Autodesk Inventor part; units mm, degrees
ref_plane "Work Plane5" through (4.6312, 3.8939, 0) normal (1, 0, 0) x (0, 0, -1)
ref_plane "YZ Plane" through (0, 0, 0) normal (1, 0, 0) x (0, 1, 0)
ref_plane "XZ Plane" through (0, 0, 0) normal (0, 1, 0) x (-1, 0, 0)
sketch "Sketch1" plane through (0, 0, 0) normal (0, 0, 1) x (1, 0, 0)
  line L0 (0, 0) -> (9.3091, 0)
  line L1 (9.3091, 0) -> (9.3091, 10)
  line L2 (9.3091, 10) -> (0, 10)
  line L3 (0, 10) -> (0, 0)
  circle A0 centre (4.6631, 6.6706) radius 2.3
  circle A1 centre (4.6631, 6.6706) radius 1
  line L4 (4.6312, 3.0206) -> (4.6312, 4.3708)
  line L5 (4.6312, 8.9703) -> (4.6312, 9.9704)
  arc A2 (4.6312, 9.9704) -> (1.3632, 6.6438) centre (4.6631, 6.6706) ccw
  arc A3 (4.639, 4.4786) -> (4.6548, 4.4787) centre (4.6389, 7.7786) ccw
  arc A4 (0, 0) -> (1.3632, 6.6438) centre (-14.8677, 6.5123) ccw
  arc A5 (0, 0) -> (4.6312, 3.0206) centre (0.3336, 4.5492) ccw
  dimension "d0" = 10
  dimension "d1" = 4.6
  dimension "d2" = 2
extrude "Extrusion1" add sketch "Sketch1" along normal blind 4 contours A4 A2 L5 A0 L4 A5 L0 | L0 A5 | A0
fillet "Fillet1" radius 2 1 edges at (4.6312, 3.0206, 2)
sketch "Sketch2" plane through (0, 0, 4) normal (0, 0, 1) x (1, 0, 0)
  line L0 (4.6312, 3.4171) -> (4.6312, 4.3708)
  arc A0 (4.6312, 4.3708) -> (4.6312, 8.9703) centre (4.6631, 6.6706) ccw
  line L1 (4.6312, 8.9703) -> (4.6312, 9.9704)
  arc A1 (4.6312, 9.9704) -> (1.3632, 6.6438) centre (4.6631, 6.6706) ccw
  circle A2 centre (4.6631, 6.6706) radius 1
  circle A3 centre (4.6631, 6.6706) radius 2.3
  arc A4 (4.4253, 2.5332) -> (4.6312, 3.4171) centre (2.6312, 3.4171) ccw
  arc A5 (0, 0) -> (1.3632, 6.6438) centre (-14.8677, 6.5123) ccw
  arc A6 (0, 0) -> (4.4253, 2.5332) centre (0.3336, 4.5492) ccw
extrude "Extrusion2" cut sketch "Sketch2" against normal blind 1.3 contours A3 A0
sketch "Sketch3" plane through (0, 0, 0) normal (0, 0, -1) x (-1, 0, 0)
  arc A0 (-1.3632, 6.6438) -> (-4.6312, 9.9704) centre (-4.6631, 6.6706) ccw
  line L0 (-4.6312, 8.9703) -> (-4.6312, 9.9704)
  arc A1 (-4.6312, 8.9703) -> (-4.6312, 4.3708) centre (-4.6631, 6.6706) ccw
  line L1 (-4.6312, 3.4171) -> (-4.6312, 4.3708)
  circle A2 centre (-4.6631, 6.6706) radius 1
  circle A3 centre (-4.6631, 6.6706) radius 2.3
  arc A4 (-4.6312, 3.4171) -> (-4.4253, 2.5332) centre (-2.6312, 3.4171) ccw
  arc A5 (-4.4253, 2.5332) -> (0, 0) centre (-0.3336, 4.5492) ccw
  arc A6 (-1.3632, 6.6438) -> (0, 0) centre (14.8677, 6.5123) ccw
extrude "Extrusion3" cut sketch "Sketch3" against normal blind 1.3 contours A3 A1
ref_plane "Work Plane5" through (4.6312, 3.8939, 0) normal (1, 0, 0) x (0, 0, -1)
sketch "Sketch6" plane through (4.6312, 3.8939, 0) normal (1, 0, 0) x (0, 0, -1)
  line L0 (0, -0.4768) -> (0, 0.4768)
  line L1 (0, 0.4768) -> (-1.3, 0.4768)
  line L2 (-1.3, 0.4768) -> (-2.7, 0.4768)
  line L3 (-2.7, 0.4768) -> (-4, 0.4768)
  line L4 (-4, -0.4768) -> (-4, 0.4768)
  circle A0 centre (-2, 0.1418) radius 0.275
  line L5 (-4, -0.4768) -> (-4, 0.4768)
  line L6 (0, -0.4768) -> (-4, -0.4768)
  line L7 (0, -0.4768) -> (0, 0.4768)
  line L8 (-4, 0.4768) -> (0, 0.4768)
  line L9 (0, 0.4768) -> (0, -0.1932)
  line L10 (0, -0.1932) -> (-4, -0.1932)
  line L11 (-4, -0.1932) -> (-4, 0.4768)
  line L12 (-4, 0.4768) -> (0, -0.1932) construction
  line L13 (-4, -0.1932) -> (0, 0.4768) construction
  point P0 (0, -3.8939)
  dimension "d22" = 0.55
  dimension "d26" = 0.67
extrude "Extrusion6" cut sketch "Sketch6" against normal blind 0.475 contours A0
fillet "Fillet2" radius 0.3 1 edges at (0, 0, 2)
properties material "Liga de Nickel-Copper 400"
The model under review builds one solid part; all positions refer to its coordinate system, in mm. A direction names the side the tool comes from. Round coordinates to 2 decimals unless told otherwise and drop trailing zeros. Write each loop counter-clockwise with the first axis right and the second up, starting at its lowest first coordinate (ties: lowest second). Pieces come first, ordered by that corner, then holes. Notation, with made-up numbers: (80, -1.5) - (121, -1.5) arc R24 cw to (121, 21.5) - close; hole circle Ø5 at (86.5, 64). An arc over 180 degrees is marked (long way). Answer as CSV lines item,"result". Start each with the question number.
(1) We need section A-A on x = 5.25. State the section outline as (y, z) points.
(2) For faces 4 (the flat face through (4.631, 3.6, 2)), 5 (the flat face through (2, 4, 0)), 6 (the cylindrical face through (2.364, 6.721, 3.359)), 7 (the flat face through (4.631, 9.5, 2)), 8 (the flat face through (6, 7, 1.3)), list the 3-axis set-ups (+Z, -Z, +X, -X, +Y, -Y) from which the entire face can be reached by the end or side of a thin tool; tool diameter is ignored.
(3) We need section C-C on y = 8. State the section outline as (x, z) points, plus the area to 3 significant figures.
(4) Draft analysis for pull direction X (two halves, no side actions). For faces 1 (the cylindrical face through (4.446, 7.647, 1.99)), 2 (the flat face through (6, 6, 2.7)), 3 (the cylindrical face through (2.364, 6.62, 0.641)), state which applies: pulls with the +X half, pulls with the -X half, needs draft (parallel to the pull), parting line crosses it, or undercut.
(5) For pin 1 Ø3.5 at (x, y) = (4, 7.5) entering from +Z; pin 2 Ø1 at (x, y) = (6, 7.5) entering from +Z; pin 3 Ø2 at (y, z) = (1.5, 0.5) entering from +X, all flat-tipped, find the tip position at first contact; note any pin that passes through.
(6) We need section B-B on x = 3. State the section outline as (y, z) points.
(7) To check wall thickness, follow line 1 (Y direction, x = 4.3, z = 2); line 2 (Y direction, x = 4.4, z = 2); line 3 (Y direction, x = 4.25, z = 2.4). State the ranges of each line that lie inside material, in increasing order.
(8) We need section D-D on x = 1.75. State the section outline as (y, z) points, plus the area to 3 significant figures.
Worked answers:
1,outline,"(4.45, 1.3) - (5.86, 1.3) - (5.86, 2.7) - (4.45, 2.7) - close; (7.48, 1.3) - (8.89, 1.3) - (8.89, 2.7) - (7.48, 2.7) - close"
2,face 4,"+Z, -Z, +X, -Y"
2,face 5,"-Z, +X, -X, +Y, -Y"
2,face 6,"+Z, +X"
2,face 7,"+Z, -Z, +X, +Y"
2,face 8,"-Z, +X"
3,outline,"(1.64, 0) - (2.79, 0) - (2.79, 1.3) - (6.54, 1.3) - (6.54, 2.7) - (2.79, 2.7) - (2.79, 4) - (1.64, 4) - close"
3,area,"9.83 mm²"
4,face 1,"undercut"
4,face 2,"needs draft"
4,face 3,"pulls with the +X half"
5,pin 1,"z = 4"
5,pin 2,"z = 2.7"
5,pin 3,"x = 4.41"
6,outline,"(0.85, 0) - (5.08, 0) - (5.08, 1.3) - (8.26, 1.3) - (8.26, 0) - (9.52, 0) - (9.52, 4) - (8.26, 4) - (8.26, 2.7) - (5.08, 2.7) - (5.08, 4) - (0.85, 4) - close"
7,line 1,"2.3 to 3.76, 4.31 to 5.74, 7.6 to 9.95"
7,line 2,"2.48 to 3.76, 4.31 to 5.71, 7.64 to 9.96"
7,line 3,"2.21 to 5.76, 7.58 to 9.94"
8,outline,"(0.21, 0) - (8.22, 0) - (8.22, 4) - (0.21, 4) - close"
8,area,"32.0 mm²"
